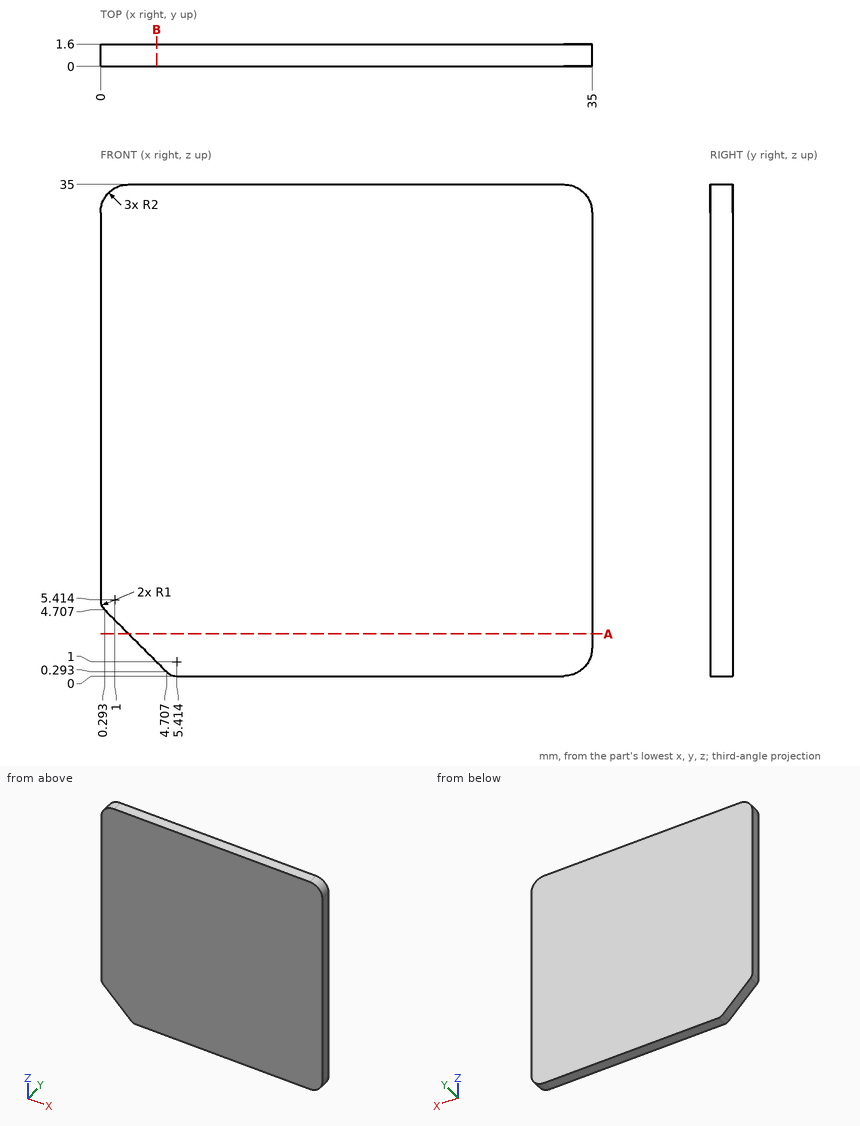
Input: dimensioned drawing with shaded views. Units: mm. Origin: part minimum x, y, z. Give positions to 0.01 mm unless a question says otherwise; leave off trailing zeros. Write each loop counter-clockwise with the first axis right and the second up, starting at its lowest first coordinate (ties: lowest second). Pieces come first, ordered by that corner, then holes. Notation, with made-up numbers: M -17.75,78 L -6.75,78 A19 ccw -6.75,95 Z; hole C 24.5,79.25 d6. An arc over 180 degrees is marked long. Return JSON: item names as keys, results as strings. Group by question number.
1) Cut plane A-A, the plane z = 3. Output: boundary loops of the cut face in (x, y), plus the area to 3 significant figures.
2) Cut plane B-B, the plane x = 4. Output: boundary loops of the cut face in (y, z).
3) Pin query (flat end, axial travel): P1, Ø4, axis at x = 15.5, z = 24, coming from the -Y side. Return the tip coordinate at first contact, or that it passes through.
4) Material intervals for line 1 along Z through (x, y) = (2, 1.1), sorted ascending. Write a range as [from, to].
Recorded:
{
 "1": {"outline": "M 2,0 L 35,0 L 35,1.6 L 2,1.6 Z", "area": "52.8 mm²"},
 "2": {"outline": "M 0,1 L 1.6,1 L 1.6,35 L 0,35 Z"},
 "3": {"P1": "stops at y = 0"},
 "4": {"line 1": "z = [3, 35]"}
}
